Read the model definition and answer for the solid it produces. Units are mm, in the model's axes. A direction names the side the tool comes from. Give positions to 0.01 mm unless a question says otherwise; leave off trailing zeros. Order: outer loops, then holes, each group sorted by start corner. A loop starts at its lowest first (then second) coordinate and runs counter-clockwise, first axis right, second up. Notation, with made-up numbers: (42.5, 67.25) - (69.5, 67.25) arc R17 ccw to (69.5, 99.25) - close; hole circle Ø10 at (-8.5, 5). An arc over 180 degrees is marked (long way). Write each question's results on one line, items separated by ' | '. Start each with the question number.
Q1. Find section D-D on z = -69. Give the vertices of the cut face in (x, y).
Q2. Find section C-C on y = -43. Give the vertices of the cut face in (x, z).
Q3. Find the intervals of material crossed by line 1 along X through (y, z) = (-40, 187); line 2 along X through (y, z) = (1, -36); line 3 along Y through (x, z) = (20.5, -53.5), in increasing order. Write a range as from..to.
Q4. Find section A-A on z = -25. Give the vertices of the cut face in (x, y).
Q5. A tool of negligible diameter and unlimited length cuts with its end or side. For faces 1 (the face through (67, 3, -109.348)), 2 (the face through (-77.21, -59.68, 217.47)), 3 (the face through (80.345, 3.84, 132.624)), from which of +Z, -Z, +X, -X, +Y, -Y can it reach the whole face along a straight path? Write none if from no direction.
Q6. Find section B-B on x = 25. Give the vertices of the cut face in (y, z).
Q7. Flat-ended cylindrical pins translate along their axes: P1, Ø7, axis at y = 2, z = 47.5, coming from the -X side; P2, Ø4, axis at y = 4, z = -129.38, coming from the -X side; P3, Ø5, axis at x = 56.5, z = -80.5, coming from the -Y side; P4, Ø7, axis at x = 65, y = 3.5, coming from the -Z side. Find the tip coordinate at first contact, or state that the pin passes through.
Q8. For a pull along X with two mould halves and no side action, classify faces 4 (the face through (-77.21, 8.17, 119.75)), 5 (the face through (-85.129, -26, 168)), 6 (the face through (80.3, 4.2, -136.5)), 7 (the face through (78.779, -29, 174)) as +X half, -X half, draft (parallel to the pull), parting line (faces both ways), or undercut.
from build123d import *

# Parameters (mm, degrees)
BOSS_EXTRUDE1_DEPTH  = 6.35
BOSS_EXTRUDE2_DEPTH  = 3.175
BOSS_EXTRUDE3_DEPTH  = 3.175
SKETCH6_R            = 3.175
CUT_EXTRUDE1_DEPTH   = 283.34881494
MIRROR4_COPY_1_DEPTH = 3.175
SKETCH7_R            = 2.54
CUT_EXTRUDE2_DEPTH   = 283.34881494


with BuildPart() as part:
    # Sketch3 → Boss-Extrude1 (new body)
    with BuildSketch(Plane(origin=(0, 0, 0), x_dir=(1, 0, 0), z_dir=(0, 1, 0))):
        Polygon((-78.779496576, 109.348374591), (-78.779496576, -109.348374591), (-55.662733102, -109.348374591), (-11.971276007, -48.703282599), (11.971276007, -48.703282599), (55.662733102, -109.348374591), (78.779496576, -109.348374591), (78.779496576, 109.348374591), (55.662733102, 109.348374591), (11.971276007, 48.703282599), (-11.971276007, 48.703282599), (-55.662733102, 109.348374591), align=None)
        Polygon((-11.971276007, 0), (-55.378618761, -59.954544833), (-55.662733102, 59.954544833), align=None, mode=Mode.SUBTRACT)
        Polygon((11.971276007, 0), (55.662733102, 59.954544833), (55.378618761, -59.954544833), align=None, mode=Mode.SUBTRACT)
    extrude(amount=BOSS_EXTRUDE1_DEPTH)

    # Sketch4 → Boss-Extrude2 (add)
    with BuildSketch(Plane(origin=(78.779496576, 0, 0), x_dir=(0, 0, -1), z_dir=(1, 0, 0))):
        with BuildLine():
            Line((-125.508834583, 11.113906265), (129.384720174, 11.113906265))
            ThreePointArc((129.384720174, 11.113906265), (136.501721079, 3.99690536), (129.384720174, -3.120095546))
            Line((129.384720174, -3.120095546), (-125.508834583, -3.120095546))
            ThreePointArc((-125.508834583, -3.120095546), (-132.625835488, 3.99690536), (-125.508834583, 11.113906265))
        make_face()
    boss_extrude2 = extrude(amount=BOSS_EXTRUDE2_DEPTH)

    # Mirror1: Boss-Extrude2 across plane
    add(boss_extrude2.mirror(Plane(origin=(0, 0, 0), x_dir=(0, 0, 1), z_dir=(1, 0, 0))))

    # Sketch5 → Boss-Extrude3 (add)
    with BuildSketch(Plane(origin=(81.954496576, 0, 0), x_dir=(0, 0, -1), z_dir=(1, 0, 0))):
        with BuildLine():
            Line((-121.468100538, -1.855701955), (-207.665903416, -61.368048827))
            ThreePointArc((-207.665903416, -61.368048827), (-217.559244776, -59.556175556), (-215.747371505, -49.662834197))
            Line((-215.747371505, -49.662834197), (-129.549568627, 9.849512675))
            ThreePointArc((-129.549568627, 9.849512675), (-119.656227268, 8.037639404), (-121.468100538, -1.855701955))
        make_face()
    boss_extrude3 = extrude(amount=BOSS_EXTRUDE3_DEPTH)

    # Sketch6 → Cut-Extrude1 (cut, through all)
    with BuildSketch(Plane(origin=(85.129496576, 0, 0), x_dir=(0, 0, -1), z_dir=(1, 0, 0))):
        with Locations((-211.706637461, -55.515441512)):
            Circle(SKETCH6_R)
    extrude(amount=-CUT_EXTRUDE1_DEPTH, mode=Mode.SUBTRACT)

    # Mirror3: Boss-Extrude3 across plane
    add(boss_extrude3.mirror(Plane(origin=(80.366996576, 0, 0), x_dir=(0, 0, 1), z_dir=(1, 0, 0))))

    # Mirror4: Boss-Extrude3 across plane
    add(boss_extrude3.mirror(Plane(origin=(0, 0, 0), x_dir=(0, 0, 1), z_dir=(1, 0, 0))))

    # Mirror4 copy 1 sketch → Mirror4 copy 1 (add)
    with BuildSketch(Plane(origin=(-78.779496576, 0, 0), x_dir=(0, 0, -1), z_dir=(1, 0, 0))):
        with BuildLine():
            Line((-121.468100538, -1.855701955), (-207.665903416, -61.368048827))
            ThreePointArc((-207.665903416, -61.368048827), (-217.559244776, -59.556175556), (-215.747371505, -49.662834197))
            Line((-215.747371505, -49.662834197), (-129.549568627, 9.849512675))
            ThreePointArc((-129.549568627, 9.849512675), (-119.656227268, 8.037639404), (-121.468100538, -1.855701955))
        make_face()
    extrude(amount=MIRROR4_COPY_1_DEPTH)

    # Sketch7 → Cut-Extrude2 (cut, through all)
    with BuildSketch(Plane(origin=(81.954496576, 0, 0), x_dir=(0, 0, -1), z_dir=(1, 0, 0))):
        with Locations((129.384720174, 3.99690536)):
            Circle(SKETCH7_R)
    extrude(amount=-CUT_EXTRUDE2_DEPTH, mode=Mode.SUBTRACT)


solid = part.part
Working result:
1) outline: (-81.95, -3.12) - (-78.78, -3.12) - (-78.78, 0) - (-26.59, 0) - (-26.59, 6.35) - (-78.78, 6.35) - (-78.78, 11.11) - (-81.95, 11.11) - close; (26.59, 0) - (78.78, 0) - (78.78, -3.12) - (81.95, -3.12) - (81.95, 11.11) - (78.78, 11.11) - (78.78, 6.35) - (26.59, 6.35) - close
2) outline: (-85.13, 181.06) - (-81.95, 181.06) - (-81.95, 206.1) - (-85.13, 206.1) - close; (-78.78, 181.06) - (-75.6, 181.06) - (-75.6, 206.1) - (-78.78, 206.1) - close; (75.6, 181.06) - (78.78, 181.06) - (78.78, 206.1) - (75.6, 206.1) - close; (81.95, 181.06) - (85.13, 181.06) - (85.13, 206.1) - (81.95, 206.1) - close
3) line 1: -85.13..-81.95, -78.78..-75.6, 75.6..78.78, 81.95..85.13 | line 2: -81.95..-55.61, -38.21..38.21, 55.61..81.95 | line 3: 0..6.35
4) outline: (-81.95, -3.12) - (-78.78, -3.12) - (-78.78, 0) - (-55.58, 0) - (-55.58, 6.35) - (-78.78, 6.35) - (-78.78, 11.11) - (-81.95, 11.11) - close; (-30.19, 0) - (30.19, 0) - (30.19, 6.35) - (-30.19, 6.35) - close; (55.58, 0) - (78.78, 0) - (78.78, -3.12) - (81.95, -3.12) - (81.95, 11.11) - (78.78, 11.11) - (78.78, 6.35) - (55.58, 6.35) - close
5) face 1: -Z, +Y, -Y | face 2: +X, -X | face 3: +Z
6) outline: (0, -66.79) - (6.35, -66.79) - (6.35, -17.88) - (0, -17.88) - close; (0, 18) - (6.35, 18) - (6.35, 66.79) - (0, 66.79) - close
7) P1: x = -81.95 | P2: through | P3: y = 0 | P4: z = -109.35
8) face 4: undercut | face 5: -X half | face 6: draft | face 7: undercut
